Can you work these out from the model? Positions are in its coordinate system, mm. A direction names the side the tool comes from. Coordinates: 2 decimals unless noted, no trailing zeros. Loops run counter-clockwise (first coordinate to the right, second up) from the corner with the lowest first, then second, coordinate; pieces in that order, holes last. Notation, with made-up numbers: M 74,36.25 L 118,36.25 A8 cw 118,40.25 Z; hole C 70.25,55.25 d9. An arc over 180 degrees is marked long. Answer as a JSON object with one key per item and string values. Group by question number.
Item 1: Which directions (+Z, -Z, +X, -X, +Y, -Y) give clear straight access to the entire face, cutting with the end or side of a thin tool? Please do faces 1 (the flat face through (13, -20.32, 11)), 2 (the flat face through (0, 17, 9.525)), 3 (the cylindrical face through (12.025, -13.881, 7.604)).
Item 2: Suppose I cut it at D-D (x = 0). Write out the boundary of the cut face in (y, z) (3 decimals), then the cut area to 3 significant figures.
Item 3: We'd pull the mould along X, two halves only. Please class faces 4 (the flat face through (-22.225, -4, 0)), 5 (the cylindrical face through (12.295, -13.881, -7.556)), 6 (the flat face through (13, -20.32, -11)), 7 (the cylindrical face through (1.363, 16.279, -0.903)): +X half, -X half, draft (parallel to the pull), parting line (faces both ways), or undercut.
Item 4: Suppose I cut it at C-C (y = -17). Write out the boundary of the cut face in (x, z).
Item 5: Suppose I cut it at A-A (x = -12.7). Write out the boundary of the cut face in (y, z) (3 decimals).
Item 6: Suppose I cut it at B-B (z = -2.5). Write out the boundary of the cut face in (x, y) (3 decimals), then the cut area to 3 significant figures.
Item 7: If I drill on line 1 (Y direction, x = 0, z = 11.05); line 2 (Y direction, x = -5, z = 1); line 3 (Y direction, x = 1.5, z = 1), over which ranges is the centre line in solid material (lowest first)?
Item 8: I'm going to push flat-ended pins straight in: pin 1 Ø4 at (x, z) = (-1.5, -12.5) entering from -Y; pin 2 Ø5 at (x, y) = (-5.5, 20) entering from +Z; pin 3 Ø3 at (y, z) = (9.5, 11.5) entering from +X. Where does each tip first touch, or does it pass through?
```python
from build123d import *

# Parameters (mm, degrees)
F0_W     = 44.45
F0_H     = 44.45
F1_DEPTH = 7.62
F2_R     = 3.1115
F3_DEPTH = 12.7
F4_R     = 6.2865
F5_DEPTH = 33.02
F6_R     = 3.81
F7_DEPTH = 12.7


with BuildPart() as f1:
    # F0 (on Front) → F1 (new body)
    with BuildSketch(Plane.XZ):
        Rectangle(F0_W, F0_H)
    extrude(amount=F1_DEPTH)

    # F2 (on face) → F3 (join)
    with BuildSketch(Plane.XZ.offset(7.62)):
        with Locations((-12.7, 10.641133)):
            Circle(F2_R)
        with Locations((12.7, 10.641133)):
            Circle(F2_R)
        with Locations((12.7, -10.641133)):
            Circle(F2_R)
        with Locations((-12.7, -10.641133)):
            Circle(F2_R)
    extrude(amount=F3_DEPTH)

    # F4 (on face) → F5 (join)
    with BuildSketch(Plane(origin=(0, 0, 0), x_dir=(-1, 0, 0), z_dir=(0, 1, 0))):
        with Locations((0, 5.233867)):
            Circle(F4_R)
    extrude(amount=F5_DEPTH)

    # F6 (on face) → F7 (cut)
    with BuildSketch(Plane.XY.offset(22.225)):
        with Locations((0, 16.51)):
            Circle(F6_R)
    extrude(amount=-F7_DEPTH, mode=Mode.SUBTRACT)


solid = f1.part
```
From the geometry:
{
 "1": {"face 1": "+Z, -Z, +X, -X, -Y", "face 2": "+Z", "face 3": "-Y"},
 "2": {"outline": "M -7.62,-22.225 L 0,-22.225 L 0,-1.053 L 33.02,-1.053 L 33.02,11.52 L 20.32,11.52 L 20.32,9.525 L 12.7,9.525 L 12.7,11.52 L 0,11.52 L 0,22.225 L -7.62,22.225 Z", "area": "739 mm2"},
 "3": {"face 4": "-X half", "face 5": "undercut", "face 6": "draft", "face 7": "parting line"},
 "4": {"outline": "C -12.7,-10.64 d6.22; C -12.7,10.64 d6.22; C 12.7,-10.64 d6.22; C 12.7,10.64 d6.22"},
 "5": {"outline": "M -20.32,-13.753 L -7.62,-13.753 L -7.62,-22.225 L 0,-22.225 L 0,22.225 L -7.62,22.225 L -7.62,13.753 L -20.32,13.753 L -20.32,7.53 L -7.62,7.53 L -7.62,-7.53 L -20.32,-7.53 Z"},
 "6": {"outline": "M -22.225,-7.62 L 22.225,-7.62 L 22.225,0 L -22.225,0 Z", "area": "339 mm2"},
 "7": {"line 1": "-7.62 to 12.7, 20.32 to 33.02", "line 2": "-7.62 to 0", "line 3": "-7.62 to 33.02"},
 "8": {"pin 1": "y = -7.62", "pin 2": "z = 10.76", "pin 3": "x = 4.1"}
}
